```python
from build123d import *

# Parameters (mm, degrees)
SKETCH1_R               = 9.525
EXTRUDE1_DEPTH          = 21.59
CUT_EXTRUDE1_DEPTH      = 10.525
CUT_EXTRUDE1_DEPTH_BACK = 10.525
CUT_EXTRUDE2_DEPTH      = 22.59


with BuildPart() as part:
    # Sketch1 → Extrude1 (new body)
    with BuildSketch(Plane(origin=(0, 0, 0), x_dir=(1, 0, 0), z_dir=(0, 1, 0))):
        with Locations(Location((0, 0, 0), (0, 0, 270))):  # turned: the seam where the file's is
            Circle(SKETCH1_R)
    extrude(amount=EXTRUDE1_DEPTH)

    # Sketch2 → Cut-Extrude1 (cut, two sides)
    with BuildSketch(Plane.XY) as cut_extrude1_sk:
        Polygon((-9.525, 21.59), (9.525, 2.54), (9.525, 21.59), align=None)
    extrude(amount=CUT_EXTRUDE1_DEPTH, mode=Mode.SUBTRACT)
    extrude(cut_extrude1_sk.sketch, amount=-CUT_EXTRUDE1_DEPTH_BACK, mode=Mode.SUBTRACT)

    # Sketch3 → Cut-Extrude2 (cut, through all)
    with BuildSketch(Plane.XZ):
        with BuildLine():
            Line((9.398, 1.550232563), (9.398, -1.550232563))
            ThreePointArc((9.398, -1.550232563), (9.525, 0), (9.398, 1.550232563))
        make_face()
    extrude(amount=-CUT_EXTRUDE2_DEPTH, mode=Mode.SUBTRACT)


solid = part.part
```
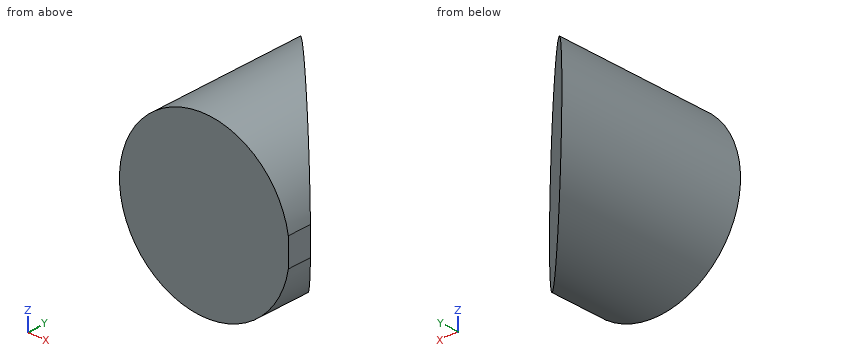
Here's how the part is built. I have some questions about the finished solid (model axes, mm). Coordinates: 2 decimals unless noted, no trailing zeros. Order: outer loops, then holes, each group sorted by start corner. A loop starts at its lowest first (then second) coordinate and runs counter-clockwise, first axis right, second up. Notation, with made-up numbers: (25, 75) - (38, 75) arc R22 ccw to (38, 92) - close; hole circle Ø5 at (-20.75, 74.25). An arc over 180 degrees is marked (long way). One line per question, with ' | ' between items. Start each with the question number.
1. Please list where these lines run through material, in increasing order: line 1 along Y through (x, z) = (-7.5, -4.25) (3 decimals); line 2 along X through (y, z) = (14, -4) (3 decimals); line 3 along Y through (x, z) = (-3.5, 4.75) (3 decimals). Write a range as [from, to].
2. If we section it at B-B (z = 0): Write out the boundary of the cut face in (x, y) (3 decimals), and give its area (3 significant figures).
3. If we section it at C-C (x = 0): Write out the boundary of the cut face in (y, z) (3 decimals).
4. If we section it at A-A (y = 3.25): Write out the boundary of the cut face in (x, z) (3 decimals), and give its area (3 significant figures).
5. I'm going to push flat-ended pins straight in: pin 1 Ø6 at (x, z) = (1.5, -1) entering from -Y; pin 2 Ø1 at (x, z) = (4, -6.5) entering from +Y (3 decimals); pin 3 Ø3 at (x, z) = (2, 5) entering from +Y (3 decimals); pin 4 Ø10 at (x, z) = (-1, 5) entering from +Y (3 decimals). Where does each tip first touch, or does it pass through?
6. If we section it at D-D (y = 7.25): Write out the boundary of the cut face in (x, z) (3 decimals).
Model answer:
1) line 1: y = [0, 19.565] | line 2: x = [-8.644, -1.935] | line 3: y = [0, 15.565]
2) outline: (-9.525, 0) - (9.398, 0) - (9.398, 2.667) - (-9.525, 21.59) - close | area: 230 mm²
3) outline: (0, -9.525) - (12.065, -9.525) - (12.065, 9.525) - (0, 9.525) - close
4) outline: (8.815, -3.609) - (8.815, 3.609) arc R9.525 ccw (long way) to start | area: 282 mm²
5) pin 1: stops at y = 0 | pin 2: stops at y = 8.565 | pin 3: stops at y = 11.565 | pin 4: stops at y = 18.065
6) outline: (4.815, -8.218) - (4.815, 8.218) arc R9.525 ccw (long way) to start
